from build123d import *

# Parameters (mm, degrees)
SKETCH1_W                      = 455
SKETCH1_H                      = 160
BOSS_EXTRUDE1_DEPTH            = 3
SKETCH2_R                      = 18
SKETCH2_R_2                    = 5
CUT_EXTRUDE1_DEPTH             = 3
F_1_16_0_0625_DIAMETER_HOLE2_D = 1.5875
CUT_EXTRUDE2_DEPTH             = 10
CUT_EXTRUDE3_DEPTH             = 10


with BuildPart() as part:
    # Sketch1 → Boss-Extrude1 (new body)
    with BuildSketch(Plane(origin=(0, 0, 0), x_dir=(1, 0, 0), z_dir=(0, 1, 0))):
        Rectangle(SKETCH1_W, SKETCH1_H)
    extrude(amount=BOSS_EXTRUDE1_DEPTH)

    # Sketch2 → Cut-Extrude1 (cut)
    with BuildSketch(Plane(origin=(0, 3, 0), x_dir=(1, 0, 0), z_dir=(0, 1, 0))):
        with Locations(Location((-167.5, 40, 0), (0, 0, 270))):
            Circle(SKETCH2_R)
        with Locations(Location((-85.151099534, 40, 0), (0, 0, 270))):
            Circle(SKETCH2_R)
        with Locations(Location((-2.651099534, 40, 0), (0, 0, 270))):
            Circle(SKETCH2_R)
        with Locations(Location((79.848900466, 39.999983289, 0), (0, 0, 270))):
            Circle(SKETCH2_R)
        with Locations(Location((162.5, 40, 0), (0, 0, 270))):
            Circle(SKETCH2_R)
        with Locations(Location((-42.5, -55, 0), (0, 0, 270))):
            Circle(SKETCH2_R_2)
        with Locations(Location((-42.5, -70, 0), (0, 0, 270))):
            Circle(SKETCH2_R_2)
        with BuildLine():
            Line((-28.777964672, -55), (-28.777964672, -73))
            ThreePointArc((-28.777964672, -73), (-23.777964672, -78), (-18.777964672, -73))
            Line((-18.777964672, -73), (-18.777964672, -55))
            ThreePointArc((-18.777964672, -55), (-23.777964672, -50), (-28.777964672, -55))
        make_face()
    extrude(amount=-CUT_EXTRUDE1_DEPTH, mode=Mode.SUBTRACT)

    # 1_16 _0.0625_ Diameter Hole2 (through all)
    with Locations(Plane(origin=(0, 3, 0), x_dir=(1, 0, 0), z_dir=(0, 1, 0))):
        with Locations((-217.5, -75), (-217.5, 70), (217.5, -70), (217.5, 65)):
            Hole(F_1_16_0_0625_DIAMETER_HOLE2_D / 2)

    # Sketch7 → Cut-Extrude2 (cut)
    with BuildSketch(Plane(origin=(0, 3, 0), x_dir=(1, 0, 0), z_dir=(0, 1, 0))):
        with BuildLine():
            ThreePointArc((-169.022220782, 57.935519058), (-167.522298342, 57.999986188), (-166.022220782, 57.939235451))
            Line((-166.022220782, 57.939235451), (-166.022220782, 66.086538462))
            Line((-166.022220782, 66.086538462), (-169.022220782, 66.086538462))
            Line((-169.022220782, 66.086538462), (-169.022220782, 57.935519058))
        make_face()
        with BuildLine():
            Line((-149.562608885, 38.5), (-141.5, 38.5))
            Line((-141.5, 38.5), (-141.5, 41.5))
            Line((-141.5, 41.5), (-149.562608885, 41.5))
            ThreePointArc((-149.562608885, 41.5), (-149.515659033, 40.750653028), (-149.5, 40))
            ThreePointArc((-149.5, 40), (-149.515659033, 39.249346972), (-149.562608885, 38.5))
        make_face()
        with BuildLine():
            Line((-193.5, 38.5), (-185.437391115, 38.5))
            ThreePointArc((-185.437391115, 38.5), (-185.5, 40), (-185.437391115, 41.5))
            Line((-185.437391115, 41.5), (-193.5, 41.5))
            Line((-193.5, 41.5), (-193.5, 38.5))
        make_face()
    extrude(amount=-CUT_EXTRUDE2_DEPTH, mode=Mode.SUBTRACT)

    # Sketch7_4 → Cut-Extrude3 (cut)
    with BuildSketch(Plane(origin=(0, 3, 0), x_dir=(1, 0, 0), z_dir=(0, 1, 0))):
        with BuildLine():
            ThreePointArc((-67.151099534, 40), (-67.166758567, 39.249346972), (-67.21370842, 38.5))
            Line((-67.21370842, 38.5), (-59.151099534, 38.5))
            Line((-59.151099534, 38.5), (-59.151099534, 41.5))
            Line((-59.151099534, 41.5), (-67.21370842, 41.5))
            ThreePointArc((-67.21370842, 41.5), (-67.166758567, 40.750653028), (-67.151099534, 40))
        make_face()
        with BuildLine():
            Line((-111.151099534, 38.5), (-103.088490649, 38.5))
            ThreePointArc((-103.088490649, 38.5), (-103.151099534, 40), (-103.088490649, 41.5))
            Line((-103.088490649, 41.5), (-111.151099534, 41.5))
            Line((-111.151099534, 41.5), (-111.151099534, 38.5))
        make_face()
        with BuildLine():
            Line((-86.651099534, 66), (-86.651099534, 57.937391115))
            ThreePointArc((-86.651099534, 57.937391115), (-85.151099534, 58), (-83.651099534, 57.937391115))
            Line((-83.651099534, 57.937391115), (-83.651099534, 66))
            Line((-83.651099534, 66), (-86.651099534, 66))
        make_face()
        with BuildLine():
            ThreePointArc((-4.151099534, 57.937391115), (-2.651099534, 58), (-1.151099534, 57.937391115))
            Line((-1.151099534, 57.937391115), (-1.151099534, 66))
            Line((-1.151099534, 66), (-4.151099534, 66))
            Line((-4.151099534, 66), (-4.151099534, 57.937391115))
        make_face()
        with BuildLine():
            Line((15.28629158, 38.5), (23.348900466, 38.5))
            Line((23.348900466, 38.5), (23.348900466, 41.5))
            Line((23.348900466, 41.5), (15.28629158, 41.5))
            ThreePointArc((15.28629158, 41.5), (15.333241433, 40.750653028), (15.348900466, 40))
            ThreePointArc((15.348900466, 40), (15.333241433, 39.249346972), (15.28629158, 38.5))
        make_face()
        with BuildLine():
            Line((-28.651099534, 38.5), (-20.588490649, 38.5))
            ThreePointArc((-20.588490649, 38.5), (-20.651099534, 40), (-20.588490649, 41.5))
            Line((-20.588490649, 41.5), (-28.651099534, 41.5))
            Line((-28.651099534, 41.5), (-28.651099534, 38.5))
        make_face()
        with BuildLine():
            ThreePointArc((78.348900466, 57.937374404), (79.848900466, 57.999983289), (81.348900466, 57.937374404))
            Line((81.348900466, 57.937374404), (81.348900466, 65.999983289))
            Line((81.348900466, 65.999983289), (78.348900466, 65.999983289))
            Line((78.348900466, 65.999983289), (78.348900466, 57.937374404))
        make_face()
        with BuildLine():
            Line((97.78629158, 38.499983289), (105.848900466, 38.499983289))
            Line((105.848900466, 38.499983289), (105.848900466, 41.499983289))
            Line((105.848900466, 41.499983289), (97.78629158, 41.499983289))
            ThreePointArc((97.78629158, 41.499983289), (97.833241433, 40.750636317), (97.848900466, 39.999983289))
            ThreePointArc((97.848900466, 39.999983289), (97.833241433, 39.249330261), (97.78629158, 38.499983289))
        make_face()
        with BuildLine():
            Line((53.848900466, 38.499983289), (61.911509351, 38.499983289))
            ThreePointArc((61.911509351, 38.499983289), (61.848900466, 39.999983289), (61.911509351, 41.499983289))
            Line((61.911509351, 41.499983289), (53.848900466, 41.499983289))
            Line((53.848900466, 41.499983289), (53.848900466, 38.499983289))
        make_face()
        with BuildLine():
            Line((136.5, 38.5), (144.562608885, 38.5))
            ThreePointArc((144.562608885, 38.5), (144.5, 40), (144.562608885, 41.5))
            Line((144.562608885, 41.5), (136.5, 41.5))
            Line((136.5, 41.5), (136.5, 38.5))
        make_face()
        with BuildLine():
            ThreePointArc((161, 57.937391115), (162.5, 58), (164, 57.937391115))
            Line((164, 57.937391115), (164, 66))
            Line((164, 66), (161, 66))
            Line((161, 66), (161, 57.937391115))
        make_face()
        with BuildLine():
            Line((180.437391115, 38.5), (188.5, 38.5))
            Line((188.5, 38.5), (188.5, 41.5))
            Line((188.5, 41.5), (180.437391115, 41.5))
            ThreePointArc((180.437391115, 41.5), (180.484340967, 40.750653028), (180.5, 40))
            ThreePointArc((180.5, 40), (180.484340967, 39.249346972), (180.437391115, 38.5))
        make_face()
    extrude(amount=-CUT_EXTRUDE3_DEPTH, mode=Mode.SUBTRACT)


solid = part.part
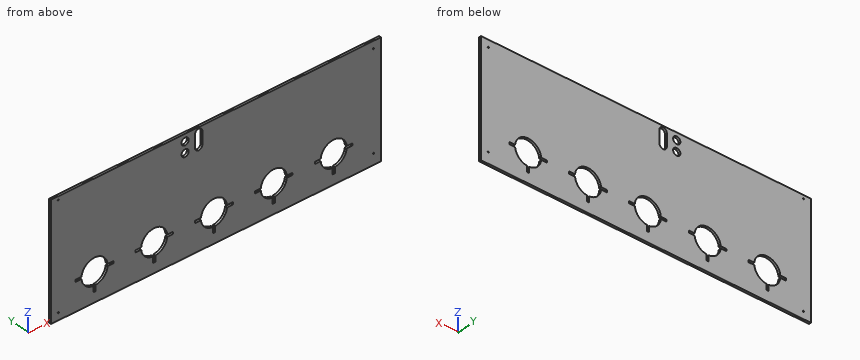
Part model, mm, in its own coordinate system. Give positions to 0.01 mm unless a question says otherwise; leave off trailing zeros. Loops run counter-clockwise (first coordinate to the right, second up) from the corner with the lowest first, then second, coordinate; pieces in that order, holes last. Notation, with made-up numbers: (-34.75, 79.25) -> (7.25, 79.25) arc R5 ccw to (7.25, 86.25) -> close; hole circle Ø4 at (-6.5, 74). An arc over 180 degrees is marked (long way). Write each question's results on one line, items separated by ' | '. Start each with the question number.
Q1. Wall check: L1, parallel to X at y = 0.75, z = 55; L2, parallel to Z at x = -24, y = 0.25; L3, parallel to Z at x = -217.5, y = 1.55. Give the ranges that are in metal, low to high.
Q2. Band-saw the part on B-B on y = 0.5. Count the separate pieces of the cut face and the enclosed holes in it, plus the area to 3 significant figures.
Q3. Pin check, flat tip, straight feed: P1, Ø9, axis at x = -42.5, z = 55, coming from the -Y side. Stop position of the tip, or through.
Q4. Band-saw the part on A-A on x = -155.5. List the corners of the cut face in (y, z).
Results are:
1) L1: x = -227.5 to -47.5, -37.5 to -28.78, -18.78 to 227.5 | L2: z = -80 to -41.5, -38.5 to 50, 78 to 80 | L3: z = -80 to -70.79, -69.21 to 74.21, 75.79 to 80
2) separate pieces: 1 | enclosed holes: 12 | area: 66,900 mm²
3) P1: passes through
4) outline: (0, -80) -> (3, -80) -> (3, -53.42) -> (0, -53.42) -> close; (0, -26.58) -> (3, -26.58) -> (3, 80) -> (0, 80) -> close
